Job drawing, mm, ordinate dimensions from the low corner. One solid piece. Round coordinates to 2 decimals unless told otherwise and drop trailing zeros. Write each loop counter-clockwise with the first axis right and the second up, starting at its lowest first coordinate (ties: lowest second). Pieces come first, ordered by that corner, then holes.
1) Saw through at C-C on x = 8.5. Write the cut outline in (y, z), and give its area (3 significant figures).
2) Saw through at B-B on y = 8. Write the cut outline in (x, z).
3) Saw through at A-A on x = 4.5. Write the cut outline in (y, z).
4) Pull direction X, two halves, no side cores. Call the marked faces 1, 2 and 3: +X half, -X half, draft (parallel to the pull), parting line (faces both ways), or undercut.
5) Flat gauge pins, fed straight in: pin 1 (1 mm diameter, centred on x = 3, y = 2, fed in from -Z); pin 2 (1.5 mm diameter, centred on x = 3, y = 6.5, fed in from +Z); pin 3 (1.5 mm diameter, centred on x = 4.5, z = 8, fed in from -Y). Where does each tip first touch, or does it go through?
6) Drill centre lines: L1, parallel to X at y = 6.5, z = 4.5; L2, parallel to Y at x = 2.5, z = 4.5. Where is each one in solid material? Low to high.
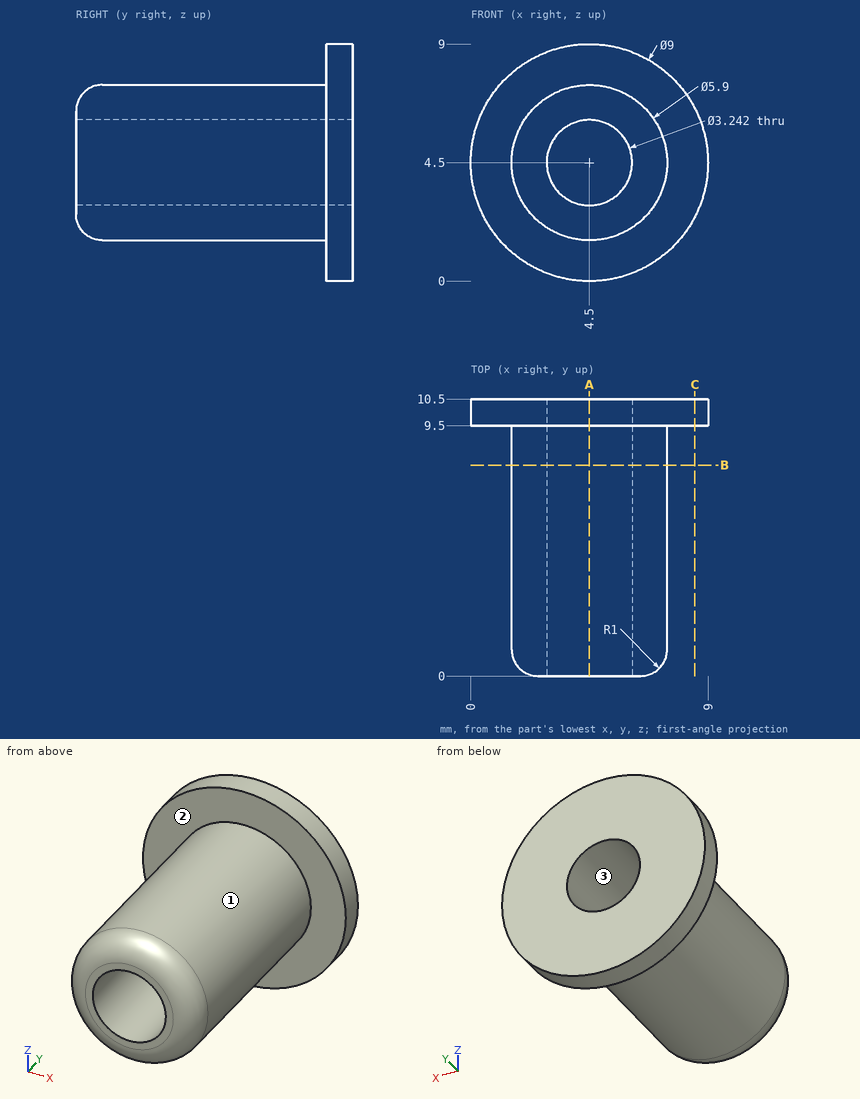
Completed:
1. outline: (9.5, 2.44) - (10.5, 2.44) - (10.5, 6.56) - (9.5, 6.56) - close
1. area: 4.12 mm2
2. outline: circle Ø5.9 at (4.5, 4.5); hole circle Ø3.24 at (4.5, 4.5)
3. outline: (0, 2.55) arc R1 ccw to (1, 1.55) - (9.5, 1.55) - (9.5, 0) - (10.5, 0) - (10.5, 2.88) - (0, 2.88) - close; (0, 6.12) - (10.5, 6.12) - (10.5, 9) - (9.5, 9) - (9.5, 7.45) - (1, 7.45) arc R1 ccw to (0, 6.45) - close
4. face 1: parting line
4. face 2: draft
4. face 3: undercut
5. pin 1: stops at z = 1.72
5. pin 2: stops at z = 7.35
5. pin 3: stops at y = 0.4
6. L1: x = 1.55 to 2.88, 6.12 to 7.45
6. L2: y = 0 to 10.5
